Work out the finished part from the listing and answer in its coordinate system (mm). A direction names the side the tool comes from. Coordinates: 2 decimals unless noted, no trailing zeros. Order: outer loops, then holes, each group sorted by start corner. A loop starts at its lowest first (then second) coordinate and runs counter-clockwise, first axis right, second up. Notation, with made-up numbers: M 28.5,87 L 80.5,87 A23 ccw 80.5,113 Z; hole C 4.5,-40 d10. An arc over 180 degrees is marked long. Use a Markdown table: item, result.
from build123d import *

# Parameters (mm, degrees)
SKIZZE1_W                                           = 135.069444444
SKIZZE1_H                                           = 100
AUFSATZ_LINEAR_AUSTRAGEN1_DEPTH                     = 123
SCHNITT_LINEAR_AUSTRAGEN1_DEPTH                     = 190.401042295
STIRNSENKUNG_F_R_M8_SENKSCHRAUBE_KOPF_B_D           = 9
STIRNSENKUNG_F_R_M8_SENKSCHRAUBE_KOPF_B_CBORE_D     = 15
STIRNSENKUNG_F_R_M8_SENKSCHRAUBE_KOPF_B_CBORE_DEPTH = 118


with BuildPart() as part:
    # Skizze1 → Aufsatz-Linear austragen1 (new body)
    with BuildSketch(Plane.XY):
        Rectangle(SKIZZE1_W, SKIZZE1_H)
    extrude(amount=AUFSATZ_LINEAR_AUSTRAGEN1_DEPTH)

    # Skizze2 → Schnitt-Linear austragen1 (cut, through all)
    with BuildSketch(Plane.ZY.offset(67.534722222)):
        Polygon((0, 11.458333333), (66.756124875, 50), (0, 71.7778768), align=None)
    extrude(amount=-SCHNITT_LINEAR_AUSTRAGEN1_DEPTH, mode=Mode.SUBTRACT)

    # Stirnsenkung für M8 Senkschraube (Kopf Button)1 (through all)
    with Locations(Plane(origin=(0, 0, 0), x_dir=(-1, 0, 0), z_dir=(0, 0, -1))):
        with Locations((-52.534722222, 0), (17.534722222, -20)):
            CounterBoreHole(STIRNSENKUNG_F_R_M8_SENKSCHRAUBE_KOPF_B_D / 2, STIRNSENKUNG_F_R_M8_SENKSCHRAUBE_KOPF_B_CBORE_D / 2, STIRNSENKUNG_F_R_M8_SENKSCHRAUBE_KOPF_B_CBORE_DEPTH)


solid = part.part
1. Section B-B on z = 103 is taken. Determine the outline of the cut face in (x, y).
Answers below:
| item | result |
|---|---|
| outline | M -67.53,-50 L 67.53,-50 L 67.53,50 L -67.53,50 Z; hole C -17.53,-20 d15; hole C 52.53,0 d15 |
2. Section D-D on x = 0 is taken. Determine the outline of the cut face in (y, z), then the cut area to 3 significant figures.
Answers below:
| item | result |
|---|---|
| outline | M -50,0 L 11.46,0 L 50,66.76 L 50,123 L -50,123 Z |
| area | 11,000 mm² |
3. For a pull along Y with two mould halves and no side action, classify faces 3 (the face through (45.38, 2.25, 58.17)), 4 (the face through (-0.95, 30.46, 32.91)), 5 (the face through (-1, 1, 123)) as +Y half, -Y half, draft (parallel to the pull), parting line (faces both ways), or undercut.
Answers below:
| item | result |
|---|---|
| face 3 | undercut |
| face 4 | +Y half |
| face 5 | draft |
4. Section C-C on x = -16 is taken. Determine the outline of the cut face in (y, z), then the cut area to 3 significant figures.
Answers below:
| item | result |
|---|---|
| outline | M -50,0 L -27.34,0 L -27.34,118 L -24.23,118 L -24.23,123 L -50,123 Z; M -15.77,118 L -12.66,118 L -12.66,0 L 11.46,0 L 50,66.76 L 50,123 L -15.77,123 Z |
| area | 9,240 mm² |
5. Section A-A on y = 0 is taken. Determine the outline of the cut face in (x, z), then the cut area to 3 significant figures.
Answers below:
| item | result |
|---|---|
| outline | M -67.53,0 L 45.03,0 L 45.03,118 L 48.03,118 L 48.03,123 L -67.53,123 Z; M 57.03,118 L 60.03,118 L 60.03,0 L 67.53,0 L 67.53,123 L 57.03,123 Z |
| area | 14,800 mm² |
6. A flat-ended cylindrical pin translates along its axis: P1, Ø13.5, axis at x = 52.53, y = 0, coming from the -Z side. Find the tip coordinate at first contact, or state that the pin passes through.
Answers below:
| item | result |
|---|---|
| P1 | z = 118 |
7. Find the intervals of material crossed by probe 1 along X at (y, z) = (-14, 16); probe 2 along Y at (x, z) = (-21, 92); probe 3 along X at (y, z) = (2.5, 41), in increasing order.
Answers below:
| item | result |
|---|---|
| probe 1 | -67.53 to -22.03, -13.03 to 67.53 |
| probe 2 | -50 to -26.65, -13.35 to 50 |
| probe 3 | -67.53 to 45.46, 59.61 to 67.53 |
8. For faces 1 (the face through (-1, 50, 94)), 2 (the face through (47.6, 0.1, 118)), determine the directions among +Z, -Z, +X, -X, +Y, -Y from which every point of the face is accessible in a straight line to the end or side of a thin tool.
Answers below:
| item | result |
|---|---|
| face 1 | +Z, -Z, +X, -X, +Y |
| face 2 | -Z |
